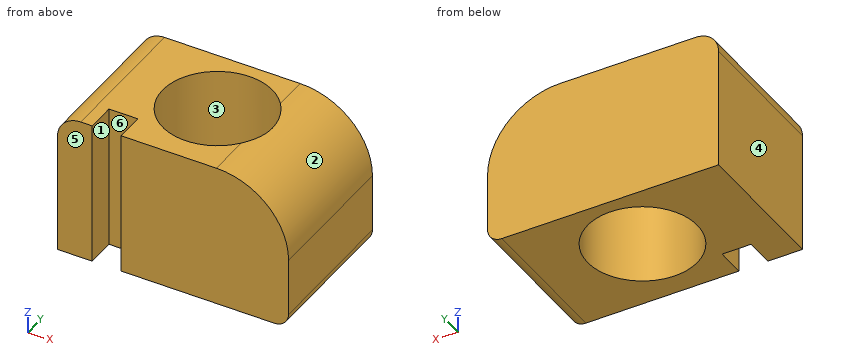
```python
from build123d import *

# Parameters (mm, degrees)
F0_W        = 80
F0_H        = 50
F0_R        = 19
F1_DEPTH    = 50
F2_T1_DEPTH = 175
F3_R        = 5
F4_R        = 8
F5_W        = 10
F5_H        = 50
F6_DEPTH    = 10


# Not quite as in the source:
# - a fillet or chamfer that OpenCascade refuses, or shapes differently, is made with other operations: its cross-section is extruded or revolved along the edge and cut away or added


with BuildPart() as f1:
    # F0 (on Top) → F1 (new body)
    with BuildSketch(Plane.XY):
        with Locations((0, -1.5042735598)):
            Rectangle(F0_W, F0_H)
        Circle(F0_R, mode=Mode.SUBTRACT)
    extrude(amount=-F1_DEPTH)

    # F2: fillet of radius 25 on 1 edges, made by hand

    # F2_s2 → F2_t1 (cut)
    with BuildSketch(Plane.XZ.offset(-85.9957264402)):
        with BuildLine():
            ThreePointArc((40, -25), (32.6776695297, -7.3223304703), (15, 0))
            Line((15, 0), (40, 0))
            Line((40, 0), (40, -25))
        make_face()
    extrude(amount=F2_T1_DEPTH, mode=Mode.SUBTRACT)

    # F3
    f3_edges = [f1.edges().sort_by_distance(p)[0] for p in [
        (40, -1.504274, -50),
    ]]
    fillet(f3_edges, radius=F3_R)

    # F4
    f4_edges = [f1.edges().sort_by_distance(p)[0] for p in [
        (-40, -1.504274, 0),
    ]]
    fillet(f4_edges, radius=F4_R)

    # F5 (on face) → F6 (cut)
    with BuildSketch(Plane.XZ.offset(26.5042735598)):
        with Locations((-23, -25)):
            Rectangle(F5_W, F5_H)
    extrude(amount=-F6_DEPTH, mode=Mode.SUBTRACT)


solid = f1.part
```
Source: CAD feature listing. Evaluate the final solid. Frame: model axes, mm. Face numbers are marked on the shaded views. A direction names the side the tool comes from. Round coordinates to 2 decimals unless told otherwise and drop trailing zeros. Loops run counter-clockwise (first coordinate to the right, second up) from the corner with the lowest first, then second, coordinate; pieces in that order, holes last. Notation, with made-up numbers: M 59.25,27.5 L 63.25,27.5 A25 cw 63.25,54.5 Z; hole C 71,52.25 d6. An arc over 180 degrees is marked long. Use a Markdown table: item, result. Add a question column.
1. Section query A-A on z = -29.5. Return the cut outline in (x, y), then the cut area to 3 significant figures.
2. Section query B-B on x = 0. Return the cut outline in (y, z).
3. Mould query, pull axis X, two halves, no side actions, for the marked faces 3, 4, 5 and 6. Classes: pulls with the +X half, pulls with the -X half, needs draft (parallel to the pull), parting line crosses it, or undercut.
4. Reachability of the marked faces 1 and 2 from +Z, -Z, +X, -X, +Y, -Y: full face, straight path, thin tool, end or side. Return the list, or none.
5. Section query D-D on y = 17. Return the cut outline in (x, z), then the cut area to 3 significant figures.
6. Section query C-C on y = 0. Return the cut outline in (x, z), then the cut area to 3 significant figures.
7. Contact query for a flat-ended pin moving along its axis: P1, Ø1, axis at x = -14.5, y = -20, coming from the +Z side. Output: stop coordinate, or through.
8. Line query: line 1 (X direction, y = 0, z = -32); line 2 (Y direction, x = 0, z = -39.5); line 3 (X direction, y = 0, z = -10). Output: solid intervals per line, ascending.
Reported:
| question | item | result |
|---|---|---|
| 1 | outline | M -40,-26.5 L -28,-26.5 L -28,-16.5 L -18,-16.5 L -18,-26.5 L 40,-26.5 L 40,23.5 L -40,23.5 Z; hole C 0,0 d38 |
| 1 | area | 2,770 mm² |
| 2 | outline | M -26.5,-50 L -19,-50 L -19,0 L -26.5,0 Z; M 19,-50 L 23.5,-50 L 23.5,0 L 19,0 Z |
| 3 | face 3 | undercut |
| 3 | face 4 | pulls with the -X half |
| 3 | face 5 | needs draft |
| 3 | face 6 | undercut |
| 4 | face 1 | +Z, -Z, -Y |
| 4 | face 2 | +Z, +X, +Y, -Y |
| 5 | outline | M -40,-50 L -8.49,-50 L -8.49,0 L -32,0 A8 ccw -40,-8 Z; M 8.49,-50 L 35,-50 A5 ccw 40,-45 L 40,-25 A25 ccw 15,0 L 8.49,0 Z |
| 5 | area | 3,000 mm² |
| 6 | outline | M -40,-50 L -19,-50 L -19,0 L -32,0 A8 ccw -40,-8 Z; M 19,-50 L 35,-50 A5 ccw 40,-45 L 40,-25 A25 ccw 19,-0.32 Z |
| 6 | area | 1,950 mm² |
| 7 | P1 | stops at z = 0 |
| 8 | line 1 | x = -40 to -19, 19 to 40 |
| 8 | line 2 | y = -26.5 to -19, 19 to 23.5 |
| 8 | line 3 | x = -40 to -19, 19 to 35 |
